Verification items for the finished model (mm, model axes). A direction names the side the tool comes from. Give positions to 0.01 mm unless a question says otherwise; leave off trailing zeros. Order: outer loops, then holes, each group sorted by start corner. A loop starts at its lowest first (then second) coordinate and runs counter-clockwise, first axis right, second up. Notation, with made-up numbers: (63, 36) -> (92, 36) arc R25 cw to (92, 59) -> close; hole circle Ø5 at (5, 47). An arc over 180 degrees is marked (long way). One line per question, with ' | ' between items. Start each with the question number.
Q1. Go/stop test with flat-tipped pins: pin 1 (7.5 mm diameter, centred on x = -125, y = -6.5, fed in from +Z) (3 decimals); pin 2 (1 mm diameter, centred on y = -6.5, z = 6, fed in from +X); pin 3 (1.5 mm diameter, centred on y = -11.5, z = 5, fed in from -X). Record where each tip stops, or that it passes through.
Q2. Access from +Z, -Z, +X, -X, +Y, -Y to the whole of each face (thin tool, end or side, straight path). Record for faces 1 (the cylindrical face through (-21.169, -13.902, 3.863)), 2 (the flat face through (-101, -13, 4.445)).
Q3. Section check C-C on x = -115. Record the cut outline in (y, z) (3 decimals).
Q4. Section check A-A on y = -12.7. Give the number of separate pieces and of enclosed holes in the cut face, plus the area to 3 significant figures.
Q5. Material ranges on probe 1 along Y at (x, z) = (-187, 5.5); probe 2 along X at (y, z) = (-18.25, 1.5); probe 3 along X at (y, z) = (-22, 2.5), recorded low to high. Write a range as [from, to].
Q6. Mould release check, pull along Y, two halves, no side actions. Record for faces 3 (the flat face through (-36.449, -13, 6)), 4 (the cylindrical face through (-13.782, -21.068, 3.863)), 5 (the cylindrical face through (-180.854, -12.421, 3.863)), 6 (the flat face through (-101, -25.4, 3)): released by +Y, released by -Y, zero draft, split by the parting line, or undercut.
from build123d import *

# Parameters (mm, degrees)
SKETCH1_R               = 12.7
BOSS_EXTRUDE1_DEPTH     = 7.62
SKETCH2_R               = 6.35
CUT_EXTRUDE1_DEPTH      = 7.62
SKETCH3_R               = 1.778
CUT_EXTRUDE2_DEPTH      = 7.62
CIRPATTERN1_COUNT       = 4
MIRROR1_COPY_1_SKETCH_R = 1.778
MIRROR1_COPY_1_DEPTH    = 7.62
MIRROR1_COPY_2_SKETCH_R = 1.778
MIRROR1_COPY_2_DEPTH    = 7.62
MIRROR1_COPY_3_SKETCH_R = 1.778
MIRROR1_COPY_3_DEPTH    = 7.62
SKETCH4_W               = 127
SKETCH4_H               = 3.175
CUT_EXTRUDE3_DEPTH      = 25.4


with BuildPart() as part:
    # Sketch1 → Boss-Extrude1 (new body)
    with BuildSketch(Plane.XY):
        with BuildLine():
            ThreePointArc((-12.7, -25.4), (-25.4, -12.7), (-12.7, 0))
            Line((-12.7, 0), (-187.198, 0))
            ThreePointArc((-187.198, 0), (-178.217743879, -3.719743879), (-174.498, -12.7))
            ThreePointArc((-174.498, -12.7), (-178.217743879, -21.680256121), (-187.198, -25.4))
            Line((-187.198, -25.4), (-12.7, -25.4))
        make_face()
        with Locations((-187.198, -12.7)):
            Circle(SKETCH1_R)
        with Locations((-12.7, -12.7)):
            Circle(SKETCH1_R)
    extrude(amount=BOSS_EXTRUDE1_DEPTH)

    # Sketch2 → Cut-Extrude1 (cut)
    with BuildSketch(Plane.XY.offset(7.62)):
        with Locations((-12.7, -12.7)):
            Circle(SKETCH2_R)
    cut_extrude1 = extrude(amount=-CUT_EXTRUDE1_DEPTH, mode=Mode.SUBTRACT)

    # Sketch3 → Cut-Extrude2 (cut)
    with BuildSketch(Plane.XY.offset(7.62)):
        with Locations((-2.921, -12.7)):
            Circle(SKETCH3_R)
    cut_extrude2 = extrude(amount=-CUT_EXTRUDE2_DEPTH, mode=Mode.SUBTRACT)

    # CirPattern1: Cut-Extrude2 ×4 about axis
    cirpattern1_axis = Axis((-12.7, -12.7, 0), (0, 0, 1))
    for i in range(1, CIRPATTERN1_COUNT):
        add(cut_extrude2.rotate(cirpattern1_axis, i * 360 / CIRPATTERN1_COUNT), mode=Mode.SUBTRACT)

    # Mirror1: Cut-Extrude1, Cut-Extrude2 across plane
    add(cut_extrude1.mirror(Plane(origin=(-99.949, 0, 0), x_dir=(0, 0, 1), z_dir=(1, 0, 0))), mode=Mode.SUBTRACT)
    add(cut_extrude2.mirror(Plane(origin=(-99.949, 0, 0), x_dir=(0, 0, 1), z_dir=(1, 0, 0))), mode=Mode.SUBTRACT)

    # Mirror1 copy 1 sketch → Mirror1 copy 1 (cut)
    with BuildSketch(Plane(origin=(-174.498, 0, 7.62), x_dir=(0, 1, 0), z_dir=(0, 0, 1))):
        with Locations((-2.921, 12.7)):
            Circle(MIRROR1_COPY_1_SKETCH_R)
    extrude(amount=-MIRROR1_COPY_1_DEPTH, mode=Mode.SUBTRACT)

    # Mirror1 copy 2 sketch → Mirror1 copy 2 (cut)
    with BuildSketch(Plane(origin=(-174.498, -25.4, 7.62), x_dir=(1, 0, 0), z_dir=(0, 0, 1))):
        with Locations((-2.921, 12.7)):
            Circle(MIRROR1_COPY_2_SKETCH_R)
    extrude(amount=-MIRROR1_COPY_2_DEPTH, mode=Mode.SUBTRACT)

    # Mirror1 copy 3 sketch → Mirror1 copy 3 (cut)
    with BuildSketch(Plane(origin=(-199.898, -25.4, 7.62), x_dir=(0, -1, 0), z_dir=(0, 0, 1))):
        with Locations((-2.921, 12.7)):
            Circle(MIRROR1_COPY_3_SKETCH_R)
    extrude(amount=-MIRROR1_COPY_3_DEPTH, mode=Mode.SUBTRACT)

    # Sketch4 → Cut-Extrude3 (cut)
    with BuildSketch(Plane.XZ.offset(25.4)):
        with Locations((-99.949, 6.0325)):
            Rectangle(SKETCH4_W, SKETCH4_H)
    extrude(amount=-CUT_EXTRUDE3_DEPTH, mode=Mode.SUBTRACT)


solid = part.part
Filled in:
1) pin 1: z = 4.445 | pin 2: x = -1.35 | pin 3: x = -199.89
2) face 1: +Z, -Z | face 2: +Z, +Y, -Y
3) outline: (-25.4, 0) -> (0, 0) -> (0, 4.445) -> (-25.4, 4.445) -> close
4) separate pieces: 7 | enclosed holes: 0 | area: 818 mm²
5) probe 1: [-25.4, -24.25], [-20.71, -19.05], [-6.35, -4.69], [-1.15, 0] | probe 2: [-198.62, -190.28], [-184.11, -15.79], [-9.61, -1.28] | probe 3: [-195.85, -188.91], [-185.49, -14.41], [-10.99, -4.05]
6) face 3: zero draft | face 4: undercut | face 5: undercut | face 6: released by -Y
